Here's how the part is built. I have some questions about the finished solid (model axes, mm). A direction names the side the tool comes from. Give positions to 0.01 mm unless a question says otherwise; leave off trailing zeros. Write each loop counter-clockwise with the first axis right and the second up, starting at its lowest first coordinate (ties: lowest second). Pieces come first, ordered by that corner, then holes. Notation, with made-up numbers: (-35, -26) - (-8, -26) arc R29 cw to (-8, -4) - close; hole circle Ø7 at (40, 49.5). An arc over 180 degrees is marked (long way). Use a Markdown table: item, result.
Autodesk Inventor part; units mm, degrees
ref_plane "YZ Plane" through (0, 0, 0) normal (1, 0, 0) x (0, 1, 0)
ref_plane "XZ Plane" through (0, 0, 0) normal (0, 1, 0) x (-1, 0, 0)
ref_plane "XY Plane" through (0, 0, 0) normal (0, 0, 1) x (1, 0, 0)
sketch "Sketch1" plane through (0, 0, 0) normal (0, 1, 0) x (-1, 0, 0)
  line L0 (-40, 7.5) -> (40, 7.5)
  line L1 (40, 7.5) -> (40, -7.5)
  line L2 (40, -7.5) -> (-40, -7.5)
  line L3 (-40, -7.5) -> (-40, 7.5)
  line L4 (-40, 7.5) -> (40, -7.5) construction
  line L5 (40, 7.5) -> (-40, -7.5) construction
  line L6 (30, 0) -> (-20, 0) construction
  line L7 (26.25, 3.75) -> (-16.25, 3.75)
  line L8 (-16.25, -3.75) -> (26.25, -3.75)
  arc A0 (26.25, -3.75) -> (26.25, 3.75) centre (26.25, 0) ccw
  arc A1 (-16.25, 3.75) -> (-16.25, -3.75) centre (-16.25, 0) ccw
  point P0 (0, 0)
  point P1 (5, 0)
  dimension "d0" = 15
  dimension "d1" = 80
  dimension "d2" = 7.5
  dimension "d3" = 50
  dimension "d4" = 10
extrude "Extrusion1" add sketch "Sketch1" along normal blind 12
sketch "Sketch2" plane through (0, 0, 0) normal (0, -1, 0) x (1, 0, 0)
  line L0 (-40, 7.5) -> (-35, 7.5)
  line L1 (-35, 7.5) -> (-35, -7.5)
  line L2 (-35, -7.5) -> (-40, -7.5)
  line L3 (-40, -7.5) -> (-40, 7.5)
  point P0 (0, 0)
  dimension "d7" = 5
extrude "Extrusion2" add sketch "Sketch2" along normal blind 3
sketch "Sketch3" plane through (0, 12, 0) normal (0, 1, 0) x (1, 0, 0)
  circle A0 centre (30, 0) radius 3
  line L0 (40, -7.5) -> (40, 7.5)
  point P0 (0, 0)
  dimension "d19" = 6
  dimension "d20" = 10
extrude "Extrusion3" cut sketch "Sketch3" against normal up to next
thread "Thread1"
properties part number "LabClamp"
Item 1: If we section it at D-D, the plane x = 30: Write out the boundary of the cut face in (y, z), plus the area to 3 significant figures.
Values:
| item | result |
|---|---|
| outline | (0, -7.5) - (12, -7.5) - (12, -3) - (0, -3) - close; (0, 3) - (12, 3) - (12, 7.5) - (0, 7.5) - close |
| area | 108 mm2 |
Item 2: If we section it at B-B, the plane y = 10.5: Write out the boundary of the cut face in (x, z).
Values:
| item | result |
|---|---|
| outline | (-40, -7.5) - (40, -7.5) - (40, 7.5) - (-40, 7.5) - close; hole (-26.25, -3.75) - (16.25, -3.75) arc R3.75 ccw to (16.25, 3.75) - (-26.25, 3.75) arc R3.75 ccw to start; hole circle Ø6 at (30, 0) |
Item 3: If we section it at A-A, the plane x = -16: Write out the boundary of the cut face in (y, z), plus the area to 3 significant figures.
Values:
| item | result |
|---|---|
| outline | (0, -7.5) - (12, -7.5) - (12, -3.75) - (0, -3.75) - close; (0, 3.75) - (12, 3.75) - (12, 7.5) - (0, 7.5) - close |
| area | 90.0 mm2 |
Item 4: I need wall thicknesses on line 1 along X through (y, z) = (6, 0); line 2 along Z through (x, y) = (-2, 6.75); line 3 along Z through (x, y) = (30, 8). Which ranges of each line are inside material? Lowest first, please. Write a range as [from, to].
Values:
| item | result |
|---|---|
| line 1 | x = [-40, -30], [20, 27], [33, 40] |
| line 2 | z = [-7.5, -3.75], [3.75, 7.5] |
| line 3 | z = [-7.5, -3], [3, 7.5] |
Item 5: Thinking about a two-plate mould opening in Z: for faces 4 (the cylindrical face through (-30, 6, 0)), 5 (the flat face through (-38, -3, 0)), 6 (the flat face through (-1, 6, -7.5)), which applies, +Z half, -Z half, draft (parallel to the pull), parting line (faces both ways), or undercut?
Values:
| item | result |
|---|---|
| face 4 | undercut |
| face 5 | draft |
| face 6 | -Z half |
Item 6: If we section it at C-C, the plane z = 0: Write out the boundary of the cut face in (x, y), plus the area to 3 significant figures.
Values:
| item | result |
|---|---|
| outline | (-40, -3) - (-35, -3) - (-35, 0) - (-30, 0) - (-30, 12) - (-40, 12) - close; (20, 0) - (27, 0) - (27, 12) - (20, 12) - close; (33, 0) - (40, 0) - (40, 12) - (33, 12) - close |
| area | 303 mm2 |
Item 7: Will this pin go through, and if not, where does the flat tip stop? pin 1 Ø4.5 at (x, z) = (-7, -2.5) entering from -Y.
Values:
| item | result |
|---|---|
| pin 1 | stops at y = 0 |
Item 8: For faces 1 (the flat face through (-5, 6, -3.75)), 2 (the flat face through (40, 6, 0)), 3 (the flat face through (-35, -1, 0)), which set-ups out of +Z, -Z, +X, -X, +Y, -Y let a thin tool reach every point of the face, with its end or its side?
Values:
| item | result |
|---|---|
| face 1 | +Y, -Y |
| face 2 | +Z, -Z, +X, +Y, -Y |
| face 3 | +Z, -Z, +X, -Y |
